Drawing for the job (mm, zero at the part's lowest x, y, z). A direction names the side the tool comes from. Give positions to 0.01 mm unless a question says otherwise; leave off trailing zeros. Order: outer loops, then holes, each group sorted by start corner. A loop starts at its lowest first (then second) coordinate and runs counter-clockwise, first axis right, second up. Notation, with made-up numbers: M -29,-34 L 16,-34 A27 cw 16,4 Z; hole C -25.75,28 d9. An arc over 180 degrees is marked long. One line per item, written item: value.
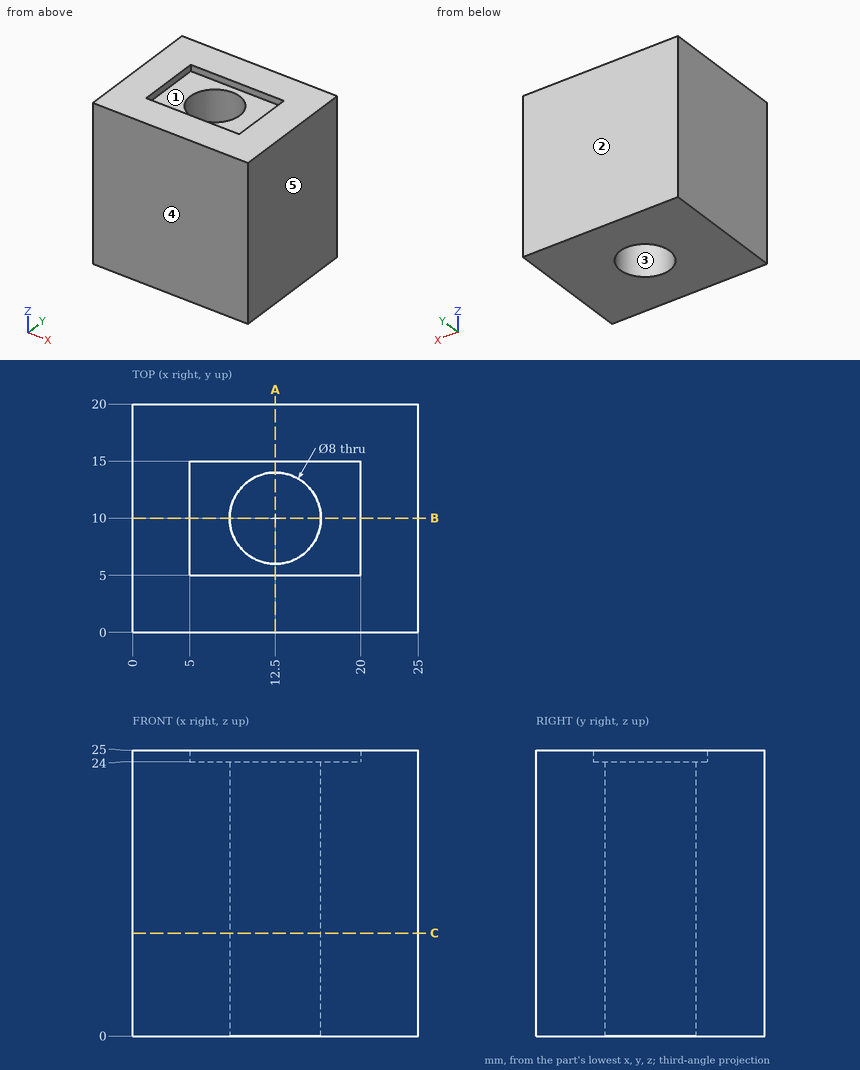
1) Saw through at A-A, the plane x = 12.5. Write the cut outline in (y, z), then the cut area to 3 significant figures.
Check values:
outline: M 0,0 L 6,0 L 6,24 L 5,24 L 5,25 L 0,25 Z; M 14,0 L 20,0 L 20,25 L 15,25 L 15,24 L 14,24 Z
area: 298 mm^2
2) Tool access for the marked faces 1 and 2: list every direction of +Z, -Z, +X, -X, +Y, -Y with a clear straight run to the whole face (end or side of a thin tool).
Check values:
face 1: +Z
face 2: +Z, -Z, +X, -X, +Y
3) Pin check, flat tips, straight feed: pin 1 (5 mm diameter, centred on x = 12.5, y = 10, fed in from +Z); pin 2 (10 mm diameter, centred on x = 8.5, z = 15.5, fed in from -Y). Stop position of each tip, or through.
Check values:
pin 1: through
pin 2: y = 0
4) Drill centre lines: probe 1 along Y at (x, z) = (12.5, 12.75); probe 2 along X at (y, z) = (10, 6); probe 3 along Y at (x, z) = (14, 21.75). Where is each one in solid material? Low to high. Write a range as from..to.
Check values:
probe 1: 0..6, 14..20
probe 2: 0..8.5, 16.5..25
probe 3: 0..6.29, 13.71..20
5) Mould opens along Y. For the marked faces 3, 4 and 5 say: released by +Y, released by -Y, zero draft, split by the parting line, or undercut.
Check values:
face 3: undercut
face 4: released by -Y
face 5: zero draft
6) Saw through at C-C, the plane z = 9. Write the cut outline in (x, y).
Check values:
outline: M 0,0 L 25,0 L 25,20 L 0,20 Z; hole C 12.5,10 d8
7) Saw through at B-B, the plane y = 10. Write the cut outline in (x, z), then the cut area to 3 significant figures.
Check values:
outline: M 0,0 L 8.5,0 L 8.5,24 L 5,24 L 5,25 L 0,25 Z; M 16.5,0 L 25,0 L 25,25 L 20,25 L 20,24 L 16.5,24 Z
area: 418 mm^2
